```python
from build123d import *

# Parameters (mm, degrees)
SKETCH2_R           = 70
BOSS_EXTRUDE1_DEPTH = 4
SKETCH8_R           = 2
CUT_EXTRUDE1_DEPTH  = 100.075728612
SKETCH34_R          = 1.5
CUT_EXTRUDE8_DEPTH  = 100.075728612
CIRPATTERN7_COUNT   = 8
SKETCH50_R          = 1.5
CUT_EXTRUDE15_DEPTH = 100.075728612
SKETCH51_R          = 1.5
CUT_EXTRUDE16_DEPTH = 100.075728612
SKETCH56_R          = 2.05
CUT_EXTRUDE19_DEPTH = 100.075728612
SKETCH57_R          = 1.5
CUT_EXTRUDE20_DEPTH = 100.075728612
CIRPATTERN13_COUNT  = 4
SKETCH60_R          = 1.5
CUT_EXTRUDE21_DEPTH = 100.075728612
CIRPATTERN14_COUNT  = 4
SKETCH49_R          = 4.5
SKETCH49_R_2        = 3.95
CUT_EXTRUDE14_DEPTH = 100.075728612
SKETCH63_R          = 1.5
CUT_EXTRUDE24_DEPTH = 100.075728612
SKETCH64_R          = 1.5
CUT_EXTRUDE25_DEPTH = 100.075728612
SKETCH65_R          = 1.5
CUT_EXTRUDE26_DEPTH = 100.075728612


with BuildPart() as part:
    # Sketch2 → Boss-Extrude1 (new body)
    with BuildSketch(Plane(origin=(0, 0, 0), x_dir=(1, 0, 0), z_dir=(0, 1, 0))):
        with Locations(Location((0, 0, 0), (0, 0, 270))):
            Circle(SKETCH2_R)
    extrude(amount=BOSS_EXTRUDE1_DEPTH)

    # Sketch8 → Cut-Extrude1 (cut, through all)
    with BuildSketch(Plane(origin=(0, 4, 0), x_dir=(1, 0, 0), z_dir=(0, 1, 0))):
        with Locations(Location((0, 0, 0), (0, 0, 270))):
            Circle(SKETCH8_R)
    extrude(amount=-CUT_EXTRUDE1_DEPTH, mode=Mode.SUBTRACT)

    # Sketch34 → Cut-Extrude8 (cut, through all)
    with BuildSketch(Plane(origin=(0, 4, 0), x_dir=(1, 0, 0), z_dir=(0, 1, 0))):
        with Locations(Location((-60.25, 0, 0), (0, 0, 270))):
            Circle(SKETCH34_R)
    cut_extrude8 = extrude(amount=-CUT_EXTRUDE8_DEPTH, mode=Mode.SUBTRACT)

    # CirPattern7: Cut-Extrude8 ×8 about axis
    cirpattern7_axis = Axis((0, 0, 0), (0, 1, 0))
    for i in range(1, CIRPATTERN7_COUNT):
        add(cut_extrude8.rotate(cirpattern7_axis, i * 360 / CIRPATTERN7_COUNT), mode=Mode.SUBTRACT)

    # Sketch50 → Cut-Extrude15 (cut, through all)
    with BuildSketch(Plane.XZ):
        with Locations(Location((-28.8, -30.5, 0), (0, 0, 270))):
            Circle(SKETCH50_R)
        with Locations(Location((-28.8, -20.5, 0), (0, 0, 270))):
            Circle(SKETCH50_R)
        with Locations(Location((54, -26, 0), (0, 0, 270))):
            Circle(SKETCH50_R)
        with Locations(Location((54, -16, 0), (0, 0, 270))):
            Circle(SKETCH50_R)
        with Locations(Location((54, 16, 0), (0, 0, 270))):
            Circle(SKETCH50_R)
        with Locations(Location((54, 26, 0), (0, 0, 270))):
            Circle(SKETCH50_R)
    extrude(amount=-CUT_EXTRUDE15_DEPTH, mode=Mode.SUBTRACT)

    # Sketch51 → Cut-Extrude16 (cut, through all)
    with BuildSketch(Plane.XZ):
        with Locations(Location((-28.8, 19.5, 0), (0, 0, 270))):
            Circle(SKETCH51_R)
        with Locations(Location((-28.8, 35.5, 0), (0, 0, 270))):
            Circle(SKETCH51_R)
    extrude(amount=-CUT_EXTRUDE16_DEPTH, mode=Mode.SUBTRACT)

    # Sketch56 → Cut-Extrude19 (cut, through all)
    with BuildSketch(Plane(origin=(0, 4, 0), x_dir=(1, 0, 0), z_dir=(0, 1, 0))):
        with Locations(Location((0, 40, 0), (0, 0, 270))):
            Circle(SKETCH56_R)
        with Locations(Location((-40, 0, 0), (0, 0, 270))):
            Circle(SKETCH56_R)
        with Locations(Location((40, 0, 0), (0, 0, 270))):
            Circle(SKETCH56_R)
        with Locations(Location((0, -40, 0), (0, 0, 270))):
            Circle(SKETCH56_R)
    extrude(amount=-CUT_EXTRUDE19_DEPTH, mode=Mode.SUBTRACT)

    # Sketch57 → Cut-Extrude20 (cut, through all)
    with BuildSketch(Plane(origin=(0, 4, 0), x_dir=(1, 0, 0), z_dir=(0, 1, 0))):
        with Locations(Location((-36.371259829, -5.986004074, 0), (0, 0, 270))):
            Circle(SKETCH57_R)
        with Locations(Location((-46.998401681, -0.149579135, 0), (0, 0, 270))):
            Circle(SKETCH57_R)
        with Locations(Location((-36.63033849, 6.135583209, 0), (0, 0, 270))):
            Circle(SKETCH57_R)
    cut_extrude20 = extrude(amount=-CUT_EXTRUDE20_DEPTH, mode=Mode.SUBTRACT)

    # CirPattern13: Cut-Extrude20 ×4 about axis
    cirpattern13_axis = Axis((0, 0, 0), (0, 1, 0))
    for i in range(1, CIRPATTERN13_COUNT):
        add(cut_extrude20.rotate(cirpattern13_axis, i * 360 / CIRPATTERN13_COUNT), mode=Mode.SUBTRACT)

    # Sketch60 → Cut-Extrude21 (cut, through all)
    with BuildSketch(Plane(origin=(0, 4, 0), x_dir=(1, 0, 0), z_dir=(0, 1, 0))):
        with Locations(Location((22, 0, 0), (0, 0, 270))):
            Circle(SKETCH60_R)
    cut_extrude21 = extrude(amount=-CUT_EXTRUDE21_DEPTH, mode=Mode.SUBTRACT)

    # CirPattern14: Cut-Extrude21 ×4 about axis
    cirpattern14_axis = Axis((0, 0, 0), (0, 1, 0))
    for i in range(1, CIRPATTERN14_COUNT):
        add(cut_extrude21.rotate(cirpattern14_axis, i * 360 / CIRPATTERN14_COUNT), mode=Mode.SUBTRACT)

    # Sketch49 → Cut-Extrude14 (cut, through all)
    with BuildSketch(Plane.XZ):
        with Locations(Location((31.205728641, 17.95, 0), (0, 0, 270))):
            Circle(SKETCH49_R)
        with Locations(Location((31.205728641, -17.95, 0), (0, 0, 270))):
            Circle(SKETCH49_R)
        with Locations(Location((-23.140353949, 27.577599952, 0), (0, 0, 270))):
            Circle(SKETCH49_R_2)
    extrude(amount=-CUT_EXTRUDE14_DEPTH, mode=Mode.SUBTRACT)

    # Sketch63 → Cut-Extrude24 (cut, through all)
    with BuildSketch(Plane.XZ):
        with Locations(Location((22.705728641, -17.95, 0), (0, 0, 270))):
            Circle(SKETCH63_R)
        with Locations(Location((39.705728641, -17.95, 0), (0, 0, 270))):
            Circle(SKETCH63_R)
        with Locations(Location((22.705728641, 17.95, 0), (0, 0, 270))):
            Circle(SKETCH63_R)
        with Locations(Location((39.705728641, 17.95, 0), (0, 0, 270))):
            Circle(SKETCH63_R)
    extrude(amount=-CUT_EXTRUDE24_DEPTH, mode=Mode.SUBTRACT)

    # Sketch64 → Cut-Extrude25 (cut, through all)
    with BuildSketch(Plane.XZ):
        with Locations(Location((4.805728641, -57, 0), (0, 0, 270))):
            Circle(SKETCH64_R)
        with Locations(Location((4.805728641, -51, 0), (0, 0, 270))):
            Circle(SKETCH64_R)
        with Locations(Location((4.805728641, 51, 0), (0, 0, 270))):
            Circle(SKETCH64_R)
        with Locations(Location((4.805728641, 57, 0), (0, 0, 270))):
            Circle(SKETCH64_R)
    extrude(amount=-CUT_EXTRUDE25_DEPTH, mode=Mode.SUBTRACT)

    # Sketch65 → Cut-Extrude26 (cut, through all)
    with BuildSketch(Plane.XZ):
        with Locations(Location((54, -30, 0), (0, 0, 270))):
            Circle(SKETCH65_R)
        with Locations(Location((54, -20, 0), (0, 0, 270))):
            Circle(SKETCH65_R)
    extrude(amount=-CUT_EXTRUDE26_DEPTH, mode=Mode.SUBTRACT)


solid = part.part
```
Part model, mm, in its own coordinate system. Round coordinates to 2 decimals unless told otherwise and drop trailing zeros. Use a Markdown table: item, result.
1) Cut at A-A, the plane y = 2. State how many separate pieces and enclosed holes the cut face has, and give its area (3 significant figures).
The answers:
| item | result |
|---|---|
| separate pieces | 1 |
| enclosed holes | 50 |
| area | 14,900 mm2 |
2) Pull direction Z, two halves, no side cores. Call faces 1 (the flat face through (-15, 4, -1)), 2 (the cylindrical face through (-26.996, 1.972, 28.434)): pulls with the +Z half, pulls with the -Z half, needs draft (parallel to the pull), parting line crosses it, or undercut.
The answers:
| item | result |
|---|---|
| face 1 | needs draft |
| face 2 | undercut |
3) Probe line 1 (Z direction, x = -42.5, y = 1.8); line 2 (X direction, y = 1.35, z = -17.95); line 3 (X direction, y = 0.3, z = -51). List the from-to ranges inside material, lowest first. Write a range as [from, to].
The answers:
| item | result |
|---|---|
| line 1 | z = [-55.62, -44.1], [-41.11, 41.11], [44.1, 55.62] |
| line 2 | x = [-67.66, 21.21], [24.21, 26.71], [35.71, 38.21], [41.21, 67.66] |
| line 3 | x = [-47.95, 3.31], [6.31, 47.95] |
4) Drop a flat-ended pin along its axis: pin 1 Ø2 at (x, y) = (-36.5, 1) entering from -Z. Give the stop position or say it passes through.
The answers:
| item | result |
|---|---|
| pin 1 | stops at z = -60.33 |
